Geometry: final body of the model. Coordinates: model frame, mm. A direction names the side the tool comes from. Coordinates: 2 decimals unless noted, no trailing zeros. Write each loop counter-clockwise with the first axis right and the second up, starting at its lowest first coordinate (ties: lowest second). Pieces come first, ordered by that corner, then holes.
from build123d import *

# Parameters (mm, degrees)
SKETCH1_R           = 76.2
SKETCH1_R_2         = 63.5
BOSS_EXTRUDE1_DEPTH = 12.7
SKETCH2_R           = 66.675
CUT_EXTRUDE1_DEPTH  = 1.5875
SKETCH3_R           = 69.85
CUT_EXTRUDE2_DEPTH  = 1.5875


with BuildPart() as part:
    # Sketch1 → Boss-Extrude1 (new, symmetric)
    with BuildSketch(Plane.XY):
        Circle(SKETCH1_R)
        Circle(SKETCH1_R_2, mode=Mode.SUBTRACT)
    extrude(amount=BOSS_EXTRUDE1_DEPTH, both=True)

    # Sketch2 → Cut-Extrude1 (cut)
    with BuildSketch(Plane.XY.offset(12.7)):
        Circle(SKETCH2_R)
    extrude(amount=-CUT_EXTRUDE1_DEPTH, mode=Mode.SUBTRACT)

    # Sketch3 → Cut-Extrude2 (cut)
    with BuildSketch(Plane(origin=(0, 0, -12.7), x_dir=(-1, 0, 0), z_dir=(0, 0, -1))):
        Circle(SKETCH3_R)
    extrude(amount=-CUT_EXTRUDE2_DEPTH, mode=Mode.SUBTRACT)


solid = part.part
Item 1: Pull-direction query (Y, two-part tool) for faces 4 (the flat face through (59, -24, 11.112)), 5 (the cylindrical face through (-60.47, -46.367, 0.178)), 6 (the flat face through (34, -62, -12.7)); classes: released by +Y, released by -Y, zero draft, split by the parting line, or undercut.
Derived:
face 4: undercut
face 5: split by the parting line
face 6: zero draft
Item 2: Section C-C, the plane z = 4.5. Output: boundary loops of the cut face in (x, y).
Derived:
outline: circle Ø152.4 at (0, 0); hole circle Ø127 at (0, 0)
Item 3: Material intervals for probe 1 along Y at (x, z) = (0, 12.35) (3 decimals); probe 2 along Y at (x, z) = (0, 0); probe 3 along X at (y, z) = (-5.5, -0.75), sorted ascending.
Derived:
probe 1: y = -76.2 to -66.675, 66.675 to 76.2
probe 2: y = -76.2 to -63.5, 63.5 to 76.2
probe 3: x = -76 to -63.26, 63.26 to 76
Item 4: Pin query (flat end, axial travel): pin 1 (3 mm diameter, centred on y = -8.5, z = 5, fed in from -X); pin 2 (4 mm diameter, centred on y = -39, z = -6, fed in from -X); pin 3 (1.5 mm diameter, centred on x = -4, z = -2, fed in from -Y). Return the tip coordinate at first contact, or that it passes through.
Derived:
pin 1: stops at x = -75.88
pin 2: stops at x = -66.61
pin 3: stops at y = -76.13
Item 5: Set-up query: faces 1 (the cylindrical face through (63.596, 20.027, 11.917)), 2 (the flat face through (0, -67, 12.7)), 3 (the cylindrical face through (55.431, -42.503, -11.917)). Return all of +Z, -Z, +X, -X, +Y, -Y with unobstructed straight access to the full face (end or side cutting, diameter ignored); none if empty.
Derived:
face 1: +Z
face 2: +Z, +X, -X, +Y, -Y
face 3: -Z
